Read the model definition and answer for the solid it produces. Units are mm, in the model's axes. Face numbers are marked on the shaded views. A direction names the side the tool comes from. Coordinates: 2 decimals unless noted, no trailing zeros. Loops run counter-clockwise (first coordinate to the right, second up) from the corner with the lowest first, then second, coordinate; pieces in that order, holes last.
from build123d import *

# Parameters (mm, degrees)
SKETCH2_R           = 30
BOSS_EXTRUDE1_DEPTH = 300
SKETCH3_R           = 20
BOSS_EXTRUDE2_DEPTH = 210
FILLET1_R           = 2
FILLET2_R           = 2


with BuildPart() as part:
    # Sketch2 → Boss-Extrude1 (new body)
    with BuildSketch(Plane.XY):
        Circle(SKETCH2_R)
    extrude(amount=BOSS_EXTRUDE1_DEPTH)

    # Sketch3 → Boss-Extrude2 (add)
    with BuildSketch(Plane.XY.offset(300)):
        Circle(SKETCH3_R)
    extrude(amount=BOSS_EXTRUDE2_DEPTH)

    # Fillet1
    fillet1_edges = [part.edges().sort_by_distance(p)[0] for p in [
        (-20, 0, 510),
    ]]
    fillet(fillet1_edges, radius=FILLET1_R)

    # Fillet2
    fillet2_edges = [part.edges().sort_by_distance(p)[0] for p in [
        (-30, 0, 300),
    ]]
    fillet(fillet2_edges, radius=FILLET2_R)


solid = part.part
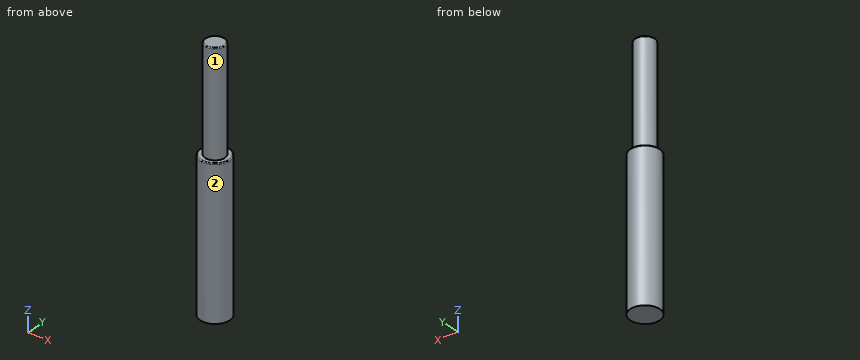
Item 1: Which of the six approach directions +Z, -Z, +X, -X, +Y, -Y give full straight-line access (tool end or side, diameter ignored) to the marked faces 1 and 2?
Numbers:
face 1: +Z
face 2: +Z, -Z
Item 2: A cutting plane is placed at A-A on x = 0. Determine the outline of the cut face in (y, z), then the cut area to 3 significant figures.
Numbers:
outline: (-30, 0) - (30, 0) - (30, 298) arc R2 ccw to (28, 300) - (20, 300) - (20, 508) arc R2 ccw to (18, 510) - (-18, 510) arc R2 ccw to (-20, 508) - (-20, 300) - (-28, 300) arc R2 ccw to (-30, 298) - close
area: 26,400 mm2
Item 3: A cutting plane is placed at C-C on z = 394.5. Determine the outline of the cut face in (x, y), then the cut area to 3 significant figures.
Numbers:
outline: circle Ø40 at (0, 0)
area: 1,260 mm2
Item 4: A cutting plane is placed at D-D on z = 128.5. Determine the outline of the cut face in (x, y).
Numbers:
outline: circle Ø60 at (0, 0)
Item 5: Given pin 1 (3 mm diameter, centred on x = 8.5, z = 398.5, fed in from +Y) (3 decimals); pin 2 (4 mm diameter, centred on x = 7.5, z = 86, fed in from +Y); pin 3 (1.5 mm diameter, centred on y = 21.5, z = 421.5, fed in from +X); pin 4 (12 mm diameter, centred on x = 2.5, z = 77.5, fed in from -Y), each flat-ended and moving along its own axis, determine where each tip first touches the part or whether it passes through.
Numbers:
pin 1: stops at y = 18.735
pin 2: stops at y = 29.49
pin 3: passes through
pin 4: stops at y = -30
Item 6: Find the intervals of material crossed by line 1 along Z through (x, y) = (-8.5, 25); line 2 along Y through (x, z) = (11, 137.5); line 3 along X through (y, z) = (10.5, 177), in increasing order.
Numbers:
line 1: z = 0 to 300
line 2: y = -27.91 to 27.91
line 3: x = -28.1 to 28.1
